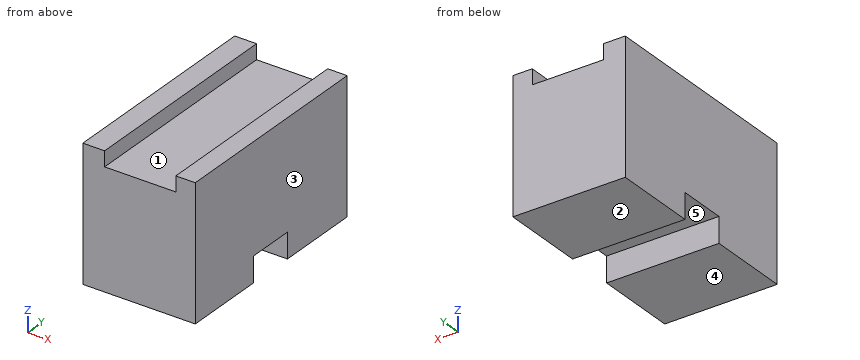
from build123d import *

# Parameters (mm, degrees)
F0_W     = 48.548784
F0_H     = 30.054009
F1_DEPTH = 25.4
F2_W     = 16.082412
F2_H     = 3.417515
F3_DEPTH = 50.8
F4_W     = 10.855629
F4_H     = 5.729359
F5_DEPTH = 50.8


with BuildPart() as f1:
    # F0 (on Right) → F1 (new body)
    with BuildSketch(Plane.YZ):
        with Locations((24.274392, 15.027004)):
            Rectangle(F0_W, F0_H)
    extrude(amount=F1_DEPTH)

    # F2 (on face) → F3 (cut)
    with BuildSketch(Plane.XZ):
        with Locations((12.966445, 28.345251)):
            Rectangle(F2_W, F2_H)
    extrude(amount=-F3_DEPTH, mode=Mode.SUBTRACT)

    # F4 (on face) → F5 (cut)
    with BuildSketch(Plane(origin=(0, 0, 0), x_dir=(0, -1, 0), z_dir=(-1, 0, 0))):
        with Locations((-24.023103, 2.864679)):
            Rectangle(F4_W, F4_H)
    extrude(amount=-F5_DEPTH, mode=Mode.SUBTRACT)


solid = f1.part
Work out the finished part from the listing and answer in its coordinate system (mm). Face numbers are marked on the shaded views. A direction names the side the tool comes from. Coordinates: 2 decimals unless noted, no trailing zeros. Write each loop counter-clockwise with the first axis right and the second up, starting at its lowest first coordinate (ties: lowest second). Pieces come first, ordered by that corner, then holes. Notation, with made-up numbers: (-28, 3) - (29, 3) arc R23 ccw to (29, 12) - close; hole circle Ø4 at (49, -37). An arc over 180 degrees is marked (long way). One line per question, with ' | ' between items.
1) Find section A-A, the plane z = 3. Determine the outline of the cut face in (x, y).
Checks:
outline: (0, 0) - (25.4, 0) - (25.4, 18.6) - (0, 18.6) - close; (0, 29.45) - (25.4, 29.45) - (25.4, 48.55) - (0, 48.55) - close
2) The mould has two halves that part along X. Classify the marked faces 1, 2 and 3: +X half, -X half, draft (parallel to the pull), parting line (faces both ways), or undercut.
Checks:
face 1: undercut | face 2: draft | face 3: +X half
3) Flat-ended cylindrical pins translate along their axes: P1, Ø5, axis at x = 13, y = 14.5, coming from the +Z side; P2, Ø1.5, axis at x = 3, y = 28, coming from the -Z side. Find the tip coordinate at first contact, or state that the pin passes through.
Checks:
P1: z = 26.64 | P2: z = 5.73
4) Find section B-B, the plane x = 4.25. Determine the outline of the cut face in (y, z).
Checks:
outline: (0, 0) - (18.6, 0) - (18.6, 5.73) - (29.45, 5.73) - (29.45, 0) - (48.55, 0) - (48.55, 30.05) - (0, 30.05) - close
5) For the marked faces 4 and 5, determine the directions among +Z, -Z, +X, -X, +Y, -Y from which every point of the face is accessible in a straight line to the end or side of a thin tool.
Checks:
face 4: -Z, +X, -X, +Y, -Y | face 5: -Z, +X, -X
6) Consider probe 1 along Y at (x, z) = (15.5, 4); probe 2 along X at (y, z) = (43, 27.5); probe 3 along Z at (x, y) = (9.5, 19.5). Determine where each line is inside the solid, lowest interval first. Write a range as [from, to].
Checks:
probe 1: [0, 18.6], [29.45, 48.55] | probe 2: [0, 4.93], [21.01, 25.4] | probe 3: [5.73, 26.64]
7) Find section C-C, the plane y = 16.5. Determine the outline of the cut face in (x, z), and give its area (3 significant figures).
Checks:
outline: (0, 0) - (25.4, 0) - (25.4, 30.05) - (21.01, 30.05) - (21.01, 26.64) - (4.93, 26.64) - (4.93, 30.05) - (0, 30.05) - close | area: 708 mm2
